Check sheet for the modelled part. Datum: model origin and axes. Units: mm. Face numbers are marked on the shaded views. A direction names the side the tool comes from. Give positions to 0.01 mm unless a question says otherwise; leave off trailing zeros. Loops run counter-clockwise (first coordinate to the right, second up) from the corner with the lowest first, then second, coordinate; pieces in that order, holes last. Notation, with made-up numbers: (60, 54) - (112, 54) arc R8 cw to (112, 65) - close; hole circle Ø10 at (-16, 24). An arc over 180 degrees is marked (long way). Use CSV: the item, a comma, the result in double quotes.
Autodesk Inventor part; units mm, degrees
ref_plane "YZ Plane" through (0, 0, 0) normal (1, 0, 0) x (0, 1, 0)
ref_plane "XZ Plane" through (0, 0, 0) normal (0, 1, 0) x (-1, 0, 0)
ref_plane "XY Plane" through (0, 0, 0) normal (0, 0, 1) x (1, 0, 0)
sketch "草圖1" plane through (0, 0, 0) normal (0, 1, 0) x (-1, 0, 0)
  line L0 (-20, 0) -> (-20, -40)
  line L1 (20, -30) -> (20, 0)
  line L2 (-20, 0) -> (20, -10)
  line L3 (-20, -10) -> (20, -20)
  arc A0 (20, 0) -> (-20, 0) centre (0, 0) ccw
  line L4 (-20, -40) -> (20, -30)
  dimension "d11" = 20
  dimension "d13" = 10
  dimension "d14" = 20
  dimension "d16" = 40
  dimension "d17" = 30
  dimension "d18" = 40
  dimension "d19" = 30
extrude "擠出1" add sketch "草圖1" along normal blind 40 contours A0 L1 L2
extrude "擠出2" add sketch "草圖1" along normal blind 30 contours L2 L1 L3 L0
extrude "擠出3" add sketch "草圖1" along normal blind 10
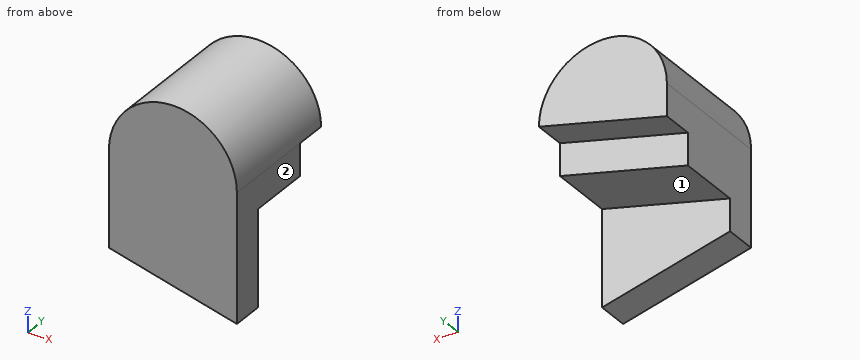
1. Scan lines: line 1 along Y through (x, z) = (-11, -14); line 2 along Y through (x, z) = (1, -34.5); line 3 along Z through (x, y) = (0, 23). Record each from-to range of solid material in increasing order.
Completed:
line 1,"y = 0 to 30"
line 2,"y = 0 to 10"
line 3,"z = -15 to 20"
2. Sectioned sample at B-B, the plane z = -2.5. Record the boundary of the cut face in (x, y), and give its area (3 significant figures).
Completed:
outline,"(-20, 0) - (20, 0) - (20, 30) - (10, 30) - (10, 40) - (-20, 40) - close"
area,"1,500 mm²"
3. Sectioned sample at C-C, the plane x = 0. Record the boundary of the cut face in (y, z), and give its area (3 significant figures).
Completed:
outline,"(0, -35) - (10, -35) - (10, -15) - (30, -15) - (30, -5) - (40, -5) - (40, 20) - (0, 20) - close"
area,"1,500 mm²"
4. Sectioned sample at A-A, the plane x = -12. Record the boundary of the cut face in (y, z).
Completed:
outline,"(0, -32) - (10, -32) - (10, -18) - (30, -18) - (30, -8) - (40, -8) - (40, 16) - (0, 16) - close"
5. Go/stop test with flat-tipped pins: pin 1 Ø4 at (x, y) = (-15, 23.5) entering from -Z; pin 2 Ø6 at (x, z) = (5, -33.5) entering from +Y; pin 3 Ø12 at (x, y) = (-8, 13.5) entering from +Z. Record where each tip stops, or that it passes through.
Completed:
pin 1,"stops at z = -19.25"
pin 2,"stops at y = 10"
pin 3,"stops at z = 19.9"
6. Set-up check for the marked faces 1 and 2: record each of +Z, -Z, +X, -X, +Y, -Y from which the full face is reachable in a straight line by a thin tool's end or side.
Completed:
face 1,"-Z, +X, +Y"
face 2,"+Z, -Z, +X, +Y, -Y"
7. Sectioned sample at D-D, the plane z = -16.5. Record the boundary of the cut face in (x, y), and give its area (3 significant figures).
Completed:
outline,"(-20, 0) - (20, 0) - (20, 10) - (-6, 10) - (-6, 30) - (-20, 30) - close"
area,"680 mm²"
